Verification items for the finished model (mm, model axes). Face numbers are marked on the shaded views. A direction names the side the tool comes from. Give positions to 0.01 mm unless a question says otherwise; leave off trailing zeros. Loops run counter-clockwise (first coordinate to the right, second up) from the corner with the lowest first, then second, coordinate; pieces in that order, holes last. Notation, with made-up numbers: M -4.5,74 L 25.5,74 A9 cw 25.5,81 Z; hole C -21,-17 d10. An arc over 180 degrees is marked long. Answer in a Markdown table with one row per item.
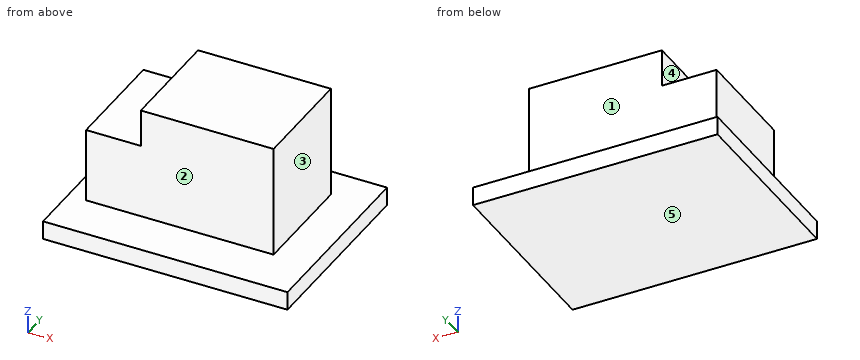
```python
from build123d import *

# Parameters (mm, degrees)
F0_W     = 34.036
F0_H     = 26.3906
F1_DEPTH = 2.5908
F2_W     = 26.1112
F2_H     = 15.1892
F3_DEPTH = 15.621
F4_W     = 7.62
F4_H     = 5.2324
F5_DEPTH = 19.7622


with BuildPart() as f1:
    # F0 (on Top) → F1 (new body)
    with BuildSketch(Plane.XY):
        Rectangle(F0_W, F0_H)
    extrude(amount=F1_DEPTH)

    # F2 (on face) → F3 (join)
    with BuildSketch(Plane.XY.offset(2.5908)):
        with Locations((-1.4478, 1.0287)):
            Rectangle(F2_W, F2_H)
    extrude(amount=F3_DEPTH)

    # F4 (on face) → F5 (cut, through all)
    with BuildSketch(Plane.XZ.offset(6.5659)):
        with Locations((-10.6934, 15.5956)):
            Rectangle(F4_W, F4_H)
    extrude(amount=-F5_DEPTH, mode=Mode.SUBTRACT)


solid = f1.part
```
Item 1: Sectioned sample at A-A (x = 1.5). Record the cut outline in (y, z).
Reported:
| item | result |
|---|---|
| outline | M -13.2,0 L 13.2,0 L 13.2,2.59 L 8.62,2.59 L 8.62,18.21 L -6.57,18.21 L -6.57,2.59 L -13.2,2.59 Z |
Item 2: Go/stop test with flat-tipped pins: pin 1 (8 mm diameter, centred on y = -4.5, z = 7, fed in from -X); pin 2 (2 mm diameter, centred on x = -7, z = 11.5, fed in from +Y); pin 3 (8.5 mm diameter, centred on x = -11.5, y = 1, fed in from +Z). Record where each tip stops, or that it passes through.
Reported:
| item | result |
|---|---|
| pin 1 | stops at x = -14.5 |
| pin 2 | stops at y = 8.62 |
| pin 3 | stops at z = 12.98 |
Item 3: Tool access check on the marked faces 1, 2, 3, 4 and 5. Record the directions out of +Z, -Z, +X, -X, +Y, -Y that give a thin tool (end or side, any length) a straight path to the whole face; none if there is none.
Reported:
| item | result |
|---|---|
| face 1 | +Z, +X, -X, +Y |
| face 2 | +Z, +X, -X, -Y |
| face 3 | +Z, +X, +Y, -Y |
| face 4 | +Z, -X, +Y, -Y |
| face 5 | -Z, +X, -X, +Y, -Y |
Item 4: Sectioned sample at C-C (z = 15). Record the cut outline in (x, y).
Reported:
| item | result |
|---|---|
| outline | M -6.88,-6.57 L 11.61,-6.57 L 11.61,8.62 L -6.88,8.62 Z |
Item 5: Sectioned sample at D-D (x = -10.5). Record the cut outline in (y, z).
Reported:
| item | result |
|---|---|
| outline | M -13.2,0 L 13.2,0 L 13.2,2.59 L 8.62,2.59 L 8.62,12.98 L -6.57,12.98 L -6.57,2.59 L -13.2,2.59 Z |
Item 6: Scan lines: L1, parallel to X at y = 3.5, z = 11; L2, parallel to Y at x = -13, z = 11.75; L3, parallel to Z at x = -15, y = -2.5. Record each from-to range of solid material in increasing order. Write a range as [from, to].
Reported:
| item | result |
|---|---|
| L1 | x = [-14.5, 11.61] |
| L2 | y = [-6.57, 8.62] |
| L3 | z = [0, 2.59] |
Item 7: Sectioned sample at B-B (y = 2.5). Record the cut outline in (x, z), and give its area (3 significant figures).
Reported:
| item | result |
|---|---|
| outline | M -17.02,0 L 17.02,0 L 17.02,2.59 L 11.61,2.59 L 11.61,18.21 L -6.88,18.21 L -6.88,12.98 L -14.5,12.98 L -14.5,2.59 L -17.02,2.59 Z |
| area | 456 mm^2 |
